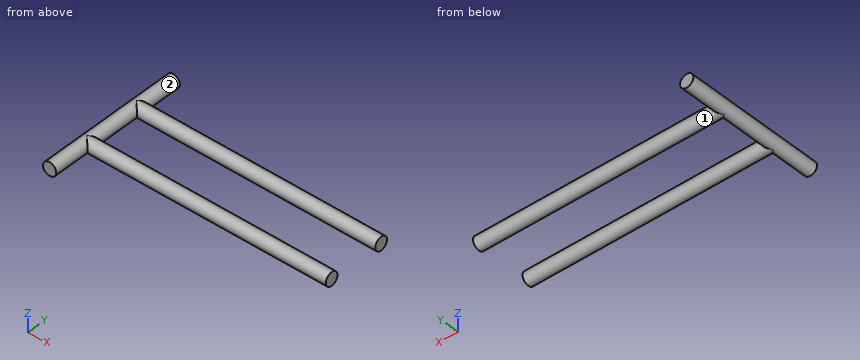
```python
from build123d import *

# Parameters (mm, degrees)
F0_R     = 2.413
F1_DEPTH = 50.8
F2_R     = 2.413
F3_DEPTH = 88.9


with BuildPart() as f1:
    # F0 (on Front) → F1 (new body)
    with BuildSketch(Plane.XZ):
        Circle(F0_R)
    extrude(amount=F1_DEPTH)

    # F2 (on Right) → F3 (join)
    with BuildSketch(Plane.YZ):
        with Locations((-35.56, 0)):
            Circle(F2_R)
        with Locations((-15.24, 0)):
            Circle(F2_R)
    extrude(amount=F3_DEPTH)


solid = f1.part
```
Verification items for the finished model (mm, model axes). Face numbers are marked on the shaded views. A direction names the side the tool comes from. Coordinates: 2 decimals unless noted, no trailing zeros. Write each loop counter-clockwise with the first axis right and the second up, starting at its lowest first coordinate (ties: lowest second). Pieces come first, ordered by that corner, then holes. Notation, with made-up numbers: (-9.5, 82) - (1.5, 82) arc R20 ccw to (1.5, 86) - close; hole circle Ø1 at (1.25, 68.5). An arc over 180 degrees is marked (long way). Write item = value, one per line.
Q1. Go/stop test with flat-tipped pins: pin 1 Ø1 at (x, z) = (53, 1.5) entering from +Y; pin 2 Ø1 at (x, z) = (19.5, 0.5) entering from -Y. Record where each tip stops, or that it passes through.
Answer:
pin_1 = -13.04
pin_2 = -37.97
Q2. Cross-section at B-B (x = 6). Enter the section's corners in (y, z).
Answer:
outline = circle Ø4.83 at (-35.56, 0); circle Ø4.83 at (-15.24, 0)
Q3. Cross-section at C-C (y = -39). Enter the section's corners in (x, z), plus the area to 3 significant figures.
Answer:
outline = circle Ø4.83 at (0, 0)
area = 18.3 mm²
Q4. Cross-section at D-D (y = -14). Enter the section's corners in (x, z).
Answer:
outline = (1.24, -2.07) - (88.9, -2.07) - (88.9, 2.07) - (1.24, 2.07) arc R2.41 ccw (long way) to start
Q5. Access from +Z, -Z, +X, -X, +Y, -Y to the whole of each face (thin tool, end or side, straight path). Record for the marked faces 1 and 2.
Answer:
face_1 = +X
face_2 = none
Q6. Material ranges on L1, parallel to Y at x = 85, z = 0.3; L2, parallel to Y at x = 32, z = 0.7; L3, parallel to Z at x = 16, y = -15.5, recorded low to high. Write a range as from..to.
Answer:
L1 = -37.95..-33.17, -17.63..-12.85
L2 = -37.87..-33.25, -17.55..-12.93
L3 = -2.4..2.4
Q7. Cross-section at A-A (z = 0). Enter the section's corners in (x, y), plus the area to 3 significant figures.
Answer:
outline = (-2.41, -50.8) - (2.41, -50.8) - (2.41, -37.97) - (88.9, -37.97) - (88.9, -33.15) - (2.41, -33.15) - (2.41, -17.65) - (88.9, -17.65) - (88.9, -12.83) - (2.41, -12.83) - (2.41, 0) - (-2.41, 0) - close
area = 1,080 mm²
